Can you work these out from the drawing? Everything is in mm from the part's minimum corner. A direction names the side the tool comes from. Round coordinates to 2 decimals unless told otherwise and drop trailing zeros. Order: outer loops, then holes, each group sorted by start corner. A loop starts at its lowest first (then second) coordinate and runs counter-clockwise, first axis right, second up. Notation, with made-up numbers: M 68,9 L 114,9 A14 ccw 114,15 Z; hole C 37,27.25 d4. An arc over 180 degrees is marked long. Write each question's results on one line, items separated by ' | '. Start each with the question number.
1. Please list where these lines run through material, in increasing order: L1, parallel to Z at x = 8.5, y = 22.5; L2, parallel to Y at x = 7, z = 7.5; L3, parallel to Y at x = 32, z = 83.5 (1 decimal).
2. Suppose I cut it at C-C on x = 50. Write out the boundary of the cut face in (y, z), and give its area (3 significant figures).
3. Suppose I cut it at D-D on z = 38.5. Write out the boundary of the cut face in (x, y), and give its area (3 significant figures).
4. We'd pull the mould along X, two halves only. Please class the marked faces 4, 5 and 6: released by +X, released by -X, zero draft, split by the parting line, or undercut.
5. I'm going to push flat-ended pins straight in: pin 1 (1 mm diameter, centred on x = 7.5, y = 31, fed in from -Z); pin 2 (1 mm diameter, centred on y = 42, z = 50.5, fed in from -X) (1 decimal); pin 3 (10 mm diameter, centred on y = 14.5, z = 53.5, fed in from -X). Where does each tip first touch, or does it pass through?
6. Suppose I cut it at A-A on z = 7.5. Write out the boundary of the cut face in (x, y), and give its area (3 significant figures).
7. Suppose I cut it at B-B on y = 4.5. Write out the boundary of the cut face in (x, z), and give its area (3 significant figures).
8. For the marked faces 1, 2 and 3, which set-ups out of +Z, -Z, +X, -X, +Y, -Y let a thin tool reach every point of the face, with its end or its side?
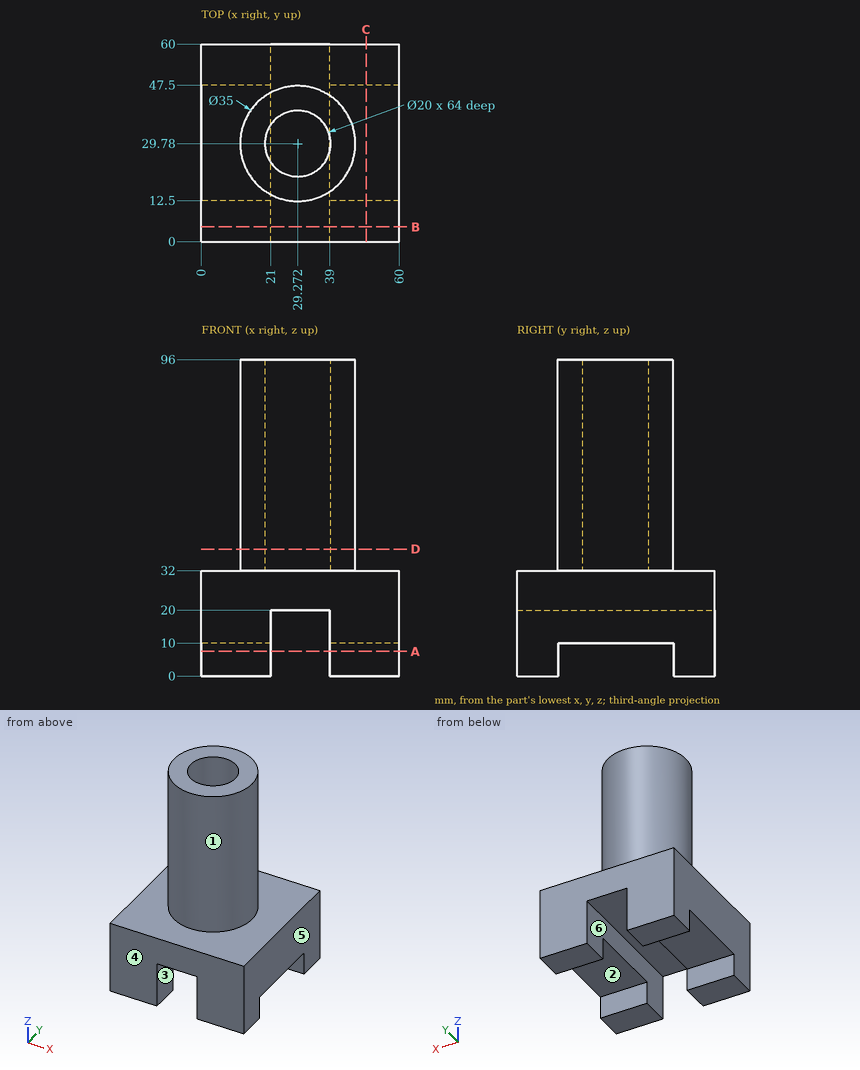
Filled sheet:
1) L1: z = 10 to 32 | L2: y = 0 to 12.5, 47.5 to 60 | L3: y = 12.5 to 20.2, 39.4 to 47.1
2) outline: M 0,0 L 12.5,0 L 12.5,10 L 47.5,10 L 47.5,0 L 60,0 L 60,32 L 0,32 Z | area: 1,570 mm^2
3) outline: C 29.27,29.78 d35; hole C 29.27,29.78 d20 | area: 648 mm^2
4) face 4: zero draft | face 5: released by +X | face 6: undercut
5) pin 1: stops at z = 10 | pin 2: stops at x = 16.3 | pin 3: stops at x = 15.11
6) outline: M 0,0 L 21,0 L 21,12.5 L 0,12.5 Z; M 0,47.5 L 21,47.5 L 21,60 L 0,60 Z; M 39,0 L 60,0 L 60,12.5 L 39,12.5 Z; M 39,47.5 L 60,47.5 L 60,60 L 39,60 Z | area: 1,050 mm^2
7) outline: M 0,0 L 21,0 L 21,20 L 39,20 L 39,0 L 60,0 L 60,32 L 0,32 Z | area: 1,560 mm^2
8) face 1: +Z | face 2: -Z, +X, -X | face 3: -Z, +Y, -Y
